Design review of the part built by this model. Coordinates are the model's own, in mm. Face numbers are marked on the shaded views. Coordinates: 2 decimals unless noted, no trailing zeros. Write each loop counter-clockwise with the first axis right and the second up, starting at its lowest first coordinate (ties: lowest second). Pieces come first, ordered by that corner, then holes. Notation, with made-up numbers: (45, 57) -> (80, 57) arc R6 ccw to (80, 68) -> close; hole circle Ø7 at (10, -3.75). An arc over 180 degrees is marked (long way). Write item = value, one per line. Start each with the question number.
```python
from build123d import *

# Parameters (mm, degrees)
F0_R      = 2.75
F1_DEPTH  = 12
F3_DEPTH  = 10.001
F4_SIZE   = 0.5
F5_SIZE   = 0.5
F6_W      = 80
F6_H      = 104
F7_DEPTH  = 5
F8_R      = 17
F8_R_2    = 5.5
F9_DEPTH  = 3
F10_R     = 5
F11_DEPTH = 7.001


with BuildPart() as f1:
    # F0 (on Right) → F1 (new body)
    with BuildSketch(Plane.YZ):
        Polygon((-80, 0), (0, 0), (80, 0), (80, 10), (40, 10), (40, 100), (0, 100), (-40, 100), (-40, 10), (-80, 10), align=None)
        with Locations((-33.2340187158, 26.7659812842)):
            Circle(F0_R, mode=Mode.SUBTRACT)
        with Locations((33.2340187158, 26.7659812842)):
            Circle(F0_R, mode=Mode.SUBTRACT)
        with Locations((-33.2340187158, 93.2340187158)):
            Circle(F0_R, mode=Mode.SUBTRACT)
        with Locations((33.2340187158, 93.2340187158)):
            Circle(F0_R, mode=Mode.SUBTRACT)
    extrude(amount=F1_DEPTH)

    # F2 (on face) → F3 (cut, through all)
    with BuildSketch(Plane.XY.offset(10)):
        with BuildLine():
            Line((10.125, 57), (10.125, 63))
            ThreePointArc((10.125, 63), (6, 67.125), (1.875, 63))
            Line((1.875, 63), (1.875, 57))
            ThreePointArc((1.875, 57), (6, 52.875), (10.125, 57))
        make_face()
        with BuildLine():
            Line((10.125, -69), (10.125, -63))
            ThreePointArc((10.125, -63), (6, -58.875), (1.875, -63))
            Line((1.875, -63), (1.875, -69))
            ThreePointArc((1.875, -69), (6, -73.125), (10.125, -69))
        make_face()
    extrude(amount=-F3_DEPTH, mode=Mode.SUBTRACT)

    # F4
    f4_edges = [f1.edges().sort_by_distance(p)[0] for p in [
        (6, 52.875, 10),
        (10.125, 57, 5),
        (6, 52.875, 0),
        (1.875, 57, 5),
        (6, -58.875, 10),
        (1.875, -63, 5),
        (6, -58.875, 0),
        (10.125, -63, 5),
    ]]
    chamfer(f4_edges, length=F4_SIZE)

    # F5
    f5_edges = [f1.edges().sort_by_distance(p)[0] for p in [
        (6, -30.484019, 93.234019),
        (0, -35.984019, 93.234019),
        (12, -35.984019, 93.234019),
        (6, 35.984019, 93.234019),
        (0, 30.484019, 93.234019),
        (12, 30.484019, 93.234019),
        (6, -30.484019, 26.765981),
        (0, -35.984019, 26.765981),
        (12, -35.984019, 26.765981),
        (6, 35.984019, 26.765981),
        (0, 30.484019, 26.765981),
        (12, 30.484019, 26.765981),
    ]]
    chamfer(f5_edges, length=F5_SIZE)

    # F6 (on face) → F7 (cut)
    with BuildSketch(Plane(origin=(0, 0, 0), x_dir=(0, -1, 0), z_dir=(-1, 0, 0))):
        with Locations((0, 48)):
            Rectangle(F6_W, F6_H)
    extrude(amount=-F7_DEPTH, mode=Mode.SUBTRACT)

    # F8 (on face) → F9 (cut)
    with BuildSketch(Plane(origin=(5, 0, 0), x_dir=(0, -1, 0), z_dir=(-1, 0, 0))):
        with Locations((0, 75)):
            Circle(F8_R)
        with Locations((0, 75)):
            Circle(F8_R_2, mode=Mode.SUBTRACT)
    extrude(amount=-F9_DEPTH, mode=Mode.SUBTRACT)

    # F10
    f10_edges = [f1.edges().sort_by_distance(p)[0] for p in [
        (8.5, 40, 10),
        (8.5, -40, 10),
    ]]
    fillet(f10_edges, radius=F10_R)

    # F11 (cut, through all): a face of the model
    f11_faces = [f1.faces().sort_by_distance(p)[0] for p in [
        (5, 0, 75),
    ]]
    extrude(f11_faces, amount=-F11_DEPTH, mode=Mode.SUBTRACT)


solid = f1.part
```
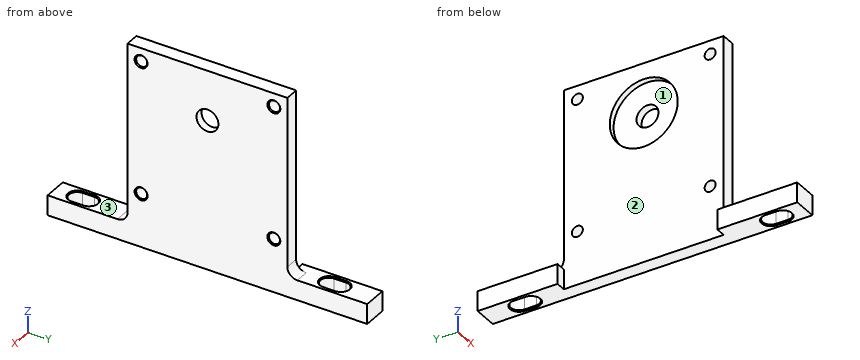
(1) Take a section at B-B, the plane z = 75. State the section outline as (x, y) points, then the cut area to 3 significant figures.
(2) Take a section at D-D, the plane y = -25.5. State the section outline as (x, z) points.
(3) Take a section at A-A, the plane y = 0. State the section outline as (x, z) points, then the cut area to 3 significant figures.
(4) Mouldability with a two-part tool opening along Z and no side actions: class the marked faces 1, 2 and 3 as pulls with the +Z half, pulls with the -Z half, needs draft (parallel to the pull), parting line crosses it, or undercut.
(5) For pin 1 Ø6 at (y, z) = (-42, 17.5) entering from -X; pin 2 Ø3.5 at (x, z) = (8.5, 39.5) entering from -Y; pin 3 Ø5.5 at (x, z) = (9.5, 56) entering from +Y, all flat-tipped, find the tip position at first contact; note any pin that passes through.
(6) For line 1 (Z direction, x = 9.75, y = 0); line 2 (X direction, y = 62.5, z = 7.5) (3 decimals); line 3 (Z direction, x = 3.25, y = -43), list the stretches that pass through material, from the lowest coordinate up.
(7) Take a section at C-C, the plane z = 60. State the section outline as (x, y) points.
Report:
q1.outline = (5, -40) -> (12, -40) -> (12, -5.5) -> (8, -5.5) -> (8, -17) -> (5, -17) -> close; (5, 17) -> (8, 17) -> (8, 5.5) -> (12, 5.5) -> (12, 40) -> (5, 40) -> close
q1.area = 414 mm2
q2.outline = (5, 0) -> (12, 0) -> (12, 100) -> (5, 100) -> close
q3.outline = (5, 0) -> (12, 0) -> (12, 69.5) -> (8, 69.5) -> (8, 58) -> (5, 58) -> close; (5, 92) -> (8, 92) -> (8, 80.5) -> (12, 80.5) -> (12, 100) -> (5, 100) -> close
q3.area = 554 mm2
q4.face_1 = undercut
q4.face_2 = needs draft
q4.face_3 = pulls with the +Z half
q5.pin_1 = 5
q5.pin_2 = -40
q5.pin_3 = 40
q6.line_1 = 0 to 69.5, 80.5 to 100
q6.line_2 = 0 to 1.875, 10.125 to 12
q6.line_3 = 0 to 10
q7.outline = (5, -40) -> (12, -40) -> (12, 40) -> (5, 40) -> (5, 8) -> (8, 8) -> (8, -8) -> (5, -8) -> close
